```python
from build123d import *

# Parameters (mm, degrees)
F1_DEPTH = 26.5
F2_R     = 6.6
F3_T     = -1.6
F4_R     = 3
F5_DEPTH = 2
F6_W     = 45.5
F6_H     = 23.3
F7_DEPTH = 2


with BuildPart() as f1:
    # F0 (on Top) → F1 (new body)
    with BuildSketch(Plane.XY):
        Polygon((29.25, 7.5), (27.65, 7.5), (-27.65, 7.5), (-29.25, 7.5), (-29.35, 7.5), (-29.35, -9.1), (-29.25, -9.1), (29.25, -9.1), (29.35, -9.1), (29.35, 7.5), align=None)
    extrude(amount=F1_DEPTH)

    # F2
    f2_edges = [f1.edges().sort_by_distance(p)[0] for p in [
        (-29.35, -9.1, 13.25),
        (29.35, -9.1, 13.25),
    ]]
    fillet(f2_edges, radius=F2_R)

    # F3
    f3_openings = [f1.faces().sort_by_distance(p)[0] for p in [
        (0, 7.5, 13.25),
    ]]
    offset(amount=F3_T, openings=f3_openings)

    # F4 (on face) → F5 (cut)
    with BuildSketch(Plane(origin=(0, 0, 0), x_dir=(1, 0, 0), z_dir=(0, 0, -1))):
        with Locations((-11.65, -0.3)):
            Circle(F4_R)
    extrude(amount=-F5_DEPTH, mode=Mode.SUBTRACT)

    # F6 (on face) → F7 (cut)
    with BuildSketch(Plane.XZ.offset(9.1)):
        with Locations((0, 13.25)):
            Rectangle(F6_W, F6_H)
    extrude(amount=-F7_DEPTH, mode=Mode.SUBTRACT)


solid = f1.part
```
Geometry: final body of the model. Coordinates: model frame, mm. A direction names the side the tool comes from. Coordinates: 2 decimals unless noted, no trailing zeros. Loops run counter-clockwise (first coordinate to the right, second up) from the corner with the lowest first, then second, coordinate; pieces in that order, holes last. Notation, with made-up numbers: (-18, 65) -> (15, 65) arc R18 ccw to (15, 74) -> close; hole circle Ø9 at (42, 19). An arc over 180 degrees is marked (long way). Use a Markdown table: item, result. Add a question column.
(1) Section query C-C, the plane z = 15. Return loops of the section in (x, y), plus the area to 3 significant figures.
(2) Line query: line 1 along X through (y, z) = (0.3, 0.4); line 2 along Y through (x, z) = (-11.65, 1.2); line 3 along Z through (x, y) = (12, 1.5). Output: solid intervals per line, ascending.
(3) Pin query (flat end, axial travel): pin 1 Ø0.8 at (y, z) = (-8, 11) entering from +X; pin 2 Ø0.5 at (y, z) = (-8.5, 15.5) entering from -X; pin 3 Ø5 at (x, z) = (-5.5, 6) entering from -Y. Return the tip coordinate at first contact, or that it passes through.
(4) Mould query, pull axis Z, two halves, no side actions, for faces 4 (the flat face through (0, -1, 1.6)), 5 (the flat face through (-29.35, 3, 13)), 6 (the flat face through (0, -1, 0)), 7 (the flat face through (-27.75, 3, 13)). Classes: pulls with the +Z half, pulls with the -Z half, needs draft (parallel to the pull), parting line crosses it, or undercut.
(5) Access query for faces 1 (the cylindrical face through (-14.647, 0.168, 0.789)), 2 (the flat face through (-22.75, -8, 13)), 3 (the cylindrical face through (26.25, -6.07, 13.41)). Directions: +Z, -Z, +X, -X, +Y, -Y. A direction counts if a zero-diameter tool reaches every point of the face in a straight line with its end or side. Return the directions, or none.
(6) Section query B-B, the plane y = 6. Return loops of the section in (x, z), plus the area to 3 significant figures.
(7) Section query A-A, the plane x = -11.65. Return loops of the section in (y, z), plus the area to 3 significant figures.
(8) Section query D-D, the plane x = 6. Return loops of the section in (y, z), plus the area to 3 significant figures.
Answer:
| question | item | result |
|---|---|---|
| 1 | outline | (-29.35, -2.5) arc R6.6 ccw to (-22.75, -9.1) -> (-22.75, -7.5) arc R5 cw to (-27.75, -2.5) -> (-27.75, 7.5) -> (-29.35, 7.5) -> close; (22.75, -9.1) arc R6.6 ccw to (29.35, -2.5) -> (29.35, 7.5) -> (27.75, 7.5) -> (27.75, -2.5) arc R5 cw to (22.75, -7.5) -> close |
| 1 | area | 61.2 mm^2 |
| 2 | line 1 | x = -29.35 to -14.65, -8.65 to 29.35 |
| 2 | line 2 | y = -9.1 to -2.7, 3.3 to 7.5 |
| 2 | line 3 | z = 0 to 1.6, 24.9 to 26.5 |
| 3 | pin 1 | stops at x = 26.94 |
| 3 | pin 2 | stops at x = -25.99 |
| 3 | pin 3 | passes through |
| 4 | face 4 | undercut |
| 4 | face 5 | needs draft |
| 4 | face 6 | pulls with the -Z half |
| 4 | face 7 | undercut |
| 5 | face 1 | -Z |
| 5 | face 2 | +Y, -Y |
| 5 | face 3 | +Y |
| 6 | outline | (-29.35, 0) -> (29.35, 0) -> (29.35, 26.5) -> (-29.35, 26.5) -> close; hole (-27.75, 1.6) -> (27.75, 1.6) -> (27.75, 24.9) -> (-27.75, 24.9) -> close |
| 6 | area | 262 mm^2 |
| 7 | outline | (-9.1, 0) -> (-2.7, 0) -> (-2.7, 1.6) -> (-9.1, 1.6) -> close; (-9.1, 24.9) -> (7.5, 24.9) -> (7.5, 26.5) -> (-9.1, 26.5) -> close; (3.3, 0) -> (7.5, 0) -> (7.5, 1.6) -> (3.3, 1.6) -> close |
| 7 | area | 43.5 mm^2 |
| 8 | outline | (-9.1, 0) -> (7.5, 0) -> (7.5, 1.6) -> (-9.1, 1.6) -> close; (-9.1, 24.9) -> (7.5, 24.9) -> (7.5, 26.5) -> (-9.1, 26.5) -> close |
| 8 | area | 53.1 mm^2 |
